Geometry: final body of the model. Coordinates: model frame, mm. A direction names the side the tool comes from. Give positions to 0.01 mm unless a question says otherwise; leave off trailing zeros. Write each loop counter-clockwise with the first axis right and the second up, starting at its lowest first coordinate (ties: lowest second). Pieces come first, ordered by that corner, then holes.
```python
from build123d import *

# Parameters (mm, degrees)
HUB_START          = -2.25
HUB_HOLE_OUTLINE_R = 0.875
HUB_HOLE_DEPTH     = 4.5


# Read off the part's stored shape, not the designer's step: Hub Hole
with BuildPart() as part:
    # Sketch3 → Revolve1 (revolve)
    with BuildSketch(Plane(origin=(0, 0, 0), x_dir=(0, 0, -1), z_dir=(1, 0, 0)), mode=Mode.PRIVATE) as revolve1_sk:
        with BuildLine():
            Line((0, 2.25), (3.25, 2.25))
            Line((3.25, 2.25), (3.25, 1.25))
            Line((3.25, 1.25), (2.5, 1.25))
            ThreePointArc((2.5, 1.25), (2.146446609, 1.103553391), (2, 0.75))
            Line((2, 0.75), (2, -0.75))
            ThreePointArc((2, -0.75), (2.146446609, -1.103553391), (2.5, -1.25))
            Line((2.5, -1.25), (3.25, -1.25))
            Line((3.25, -1.25), (3.25, -2.25))
            Line((3.25, -2.25), (0, -2.25))
            Line((0, -2.25), (0, 2.25))
        make_face()
    revolve(revolve1_sk.sketch.rotate(Axis((0, 2.25, 0), (0, -1, 0)), 180), axis=Axis((0, 2.25, 0), (0, -1, 0)))

    # Hub Hole outline → Hub Hole (cut)
    with BuildSketch(Plane(origin=(0, 0, 0), x_dir=(1, 0, 0), z_dir=(0, 1, 0)).offset(HUB_START)):
        Circle(HUB_HOLE_OUTLINE_R)
    extrude(amount=HUB_HOLE_DEPTH, mode=Mode.SUBTRACT)


solid = part.part
```
Item 1: Section C-C, the plane y = -1.4. Return the cut outline in (x, z) (3 decimals).
Found:
outline: circle Ø6.5 at (0, 0); hole circle Ø1.75 at (0, 0)
Item 2: Section B-B, the plane x = 0. Return the cut outline in (y, z) (3 decimals).
Found:
outline: (-2.25, -3.25) - (-1.25, -3.25) - (-1.25, -2.5) arc R0.5 cw to (-0.75, -2) - (0.75, -2) arc R0.5 cw to (1.25, -2.5) - (1.25, -3.25) - (2.25, -3.25) - (2.25, -0.875) - (-2.25, -0.875) - close; (-2.25, 0.875) - (2.25, 0.875) - (2.25, 3.25) - (1.25, 3.25) - (1.25, 2.5) arc R0.5 cw to (0.75, 2) - (-0.75, 2) arc R0.5 cw to (-1.25, 2.5) - (-1.25, 3.25) - (-2.25, 3.25) - close
Item 3: Reachability of faces 1 (the face through (1.978, 1.743, -2.579)), 2 (the face through (2, -1.25, -2)) from +Z, -Z, +X, -X, +Y, -Y: full face, straight path, thin tool, end or side. Return the list, or none.
Found:
face 1: +Y, -Y
face 2: none
Item 4: Line query: L1, parallel to X at y = -1.3, z = 0 (3 decimals); L2, parallel to X at y = -0.8, z = 0 (1 decimal); L3, parallel to Y at x = 0.5, z = -2.5. Output: solid intervals per line, ascending.
Found:
L1: x = -3.25 to -0.875, 0.875 to 3.25
L2: x = -2 to -0.9, 0.9 to 2
L3: y = -2.25 to -1.25, 1.25 to 2.25
Item 5: Section A-A, the plane z = 0. Return the cut outline in (x, y) (3 decimals), plus the area to 3 significant figures.
Found:
outline: (-3.25, -2.25) - (-0.875, -2.25) - (-0.875, 2.25) - (-3.25, 2.25) - (-3.25, 1.25) - (-2.5, 1.25) arc R0.5 cw to (-2, 0.75) - (-2, -0.75) arc R0.5 cw to (-2.5, -1.25) - (-3.25, -1.25) - close; (0.875, -2.25) - (3.25, -2.25) - (3.25, -1.25) - (2.5, -1.25) arc R0.5 cw to (2, -0.75) - (2, 0.75) arc R0.5 cw to (2.5, 1.25) - (3.25, 1.25) - (3.25, 2.25) - (0.875, 2.25) - close
area: 15.3 mm2
Item 6: Pin query (flat end, axial travel): pin 1 Ø1.5 at (y, z) = (-1, 1.5) entering from -X. Return the tip coordinate at first contact, or that it passes through.
Found:
pin 1: stops at x = -3.15
Item 7: Pull-direction query (Y, two-part tool) for faces 3 (the face through (2, 0, 0)), 4 (the face through (1.978, -1.757, -2.579)), 5 (the face through (1, 2.25, -1)), 6 (the face through (1, -2.25, 1)); classes: +Y half, -Y half, draft (parallel to the pull), parting line (faces both ways), or undercut.
Found:
face 3: undercut
face 4: draft
face 5: +Y half
face 6: -Y half
